Could you check a few things on this model? Use its own coordinates, in mm. A direction names the side the tool comes from. Coordinates: 2 decimals unless noted, no trailing zeros. Order: outer loops, then holes, each group sorted by start corner. A loop starts at its lowest first (then second) coordinate and runs counter-clockwise, first axis right, second up. Notation, with made-up numbers: M -8,-13.5 L -2,-13.5 A16 ccw -2,6.5 Z; hole C -15.75,32 d5. An arc over 180 degrees is marked long. Put each result on its own line as item: value. Start each with the question number.
```python
from build123d import *

# Parameters (mm, degrees)
F1_DEPTH      = 2.5
F2_R          = 1
F4_W          = 33
F4_H          = 5.5
F5_DEPTH      = 2
F5_DEPTH_BACK = 1


with BuildPart() as f1:
    # F0 (on Top) → F1 (new body)
    with BuildSketch(Plane.XY):
        Polygon((-23.6938069443, 68.3301911354), (-23.6938069443, -57.6698088646), (-10.9438069443, -57.6698088646), (-10.9438069443, -51.6698088646), (-7.9438069443, -51.6698088646), (-7.9438069443, -57.6698088646), (4.8061930557, -57.6698088646), (4.8061930557, 68.3301911354), align=None)
    extrude(amount=F1_DEPTH)

    # F2
    f2_edges = [f1.edges().sort_by_distance(p)[0] for p in [
        (-10.943807, -51.669809, 1.25),
        (-7.943807, -51.669809, 1.25),
    ]]
    fillet(f2_edges, radius=F2_R)

    # F4 (on face) → F5 (join, two sides)
    with BuildSketch(Plane(origin=(0, 67.8111465652, -5.9327065851), x_dir=(1, 0, 0), z_dir=(0, -0.9961946981, 0.0871557427))) as f5_sk:
        with Locations((-9.4438069443, 8.7053685605)):
            Rectangle(F4_W, F4_H)
    extrude(amount=-F5_DEPTH)
    extrude(f5_sk.sketch, amount=F5_DEPTH_BACK)


solid = f1.part
```
Item 1: If we section it at C-C on z = 4.15: Write out the boundary of the cut face in (x, y), then the cut area to 3 significant figures.
Item 2: I need wall thicknesses on probe 1 along Z at (x, y) = (-11, 40); probe 2 along X at (y, z) = (1.5, 1.4); probe 3 along Y at (x, z) = (-16, 3.4). Which ranges of each line are inside material? Lowest first, please.
Item 3: If we mould it in two halves opening along X, with no side actions, what happens to faces 4 (the flat face through (7.056, 69, 3)), 5 (the flat face through (-10, 6, 2.5)), 6 (the flat face through (-7.944, -55, 1))? For each: released by +X, released by -X, zero draft, split by the parting line, or undercut.
Item 4: For faces 1 (the flat face through (-10, 6, 0)), 2 (the flat face through (-23.694, 6, 1)), 3 (the flat face through (-10.944, -55, 1)), which set-ups out of +Z, -Z, +X, -X, +Y, -Y let a thin tool reach every point of the face, with its end or its side?
Item 5: If we section it at A-A on x = 3.5: Write out the boundary of the cut face in (y, z).
Item 6: For pin 1 Ø12 at (x, y) = (-12, -33) entering from +Z; pin 2 Ø2 at (y, z) = (-56.5, 1) entering from +X; pin 3 Ø0.8 at (y, z) = (-14.5, 2) entering from -X, each with a flat end and sliding along its axis, tell me the tip position at first contact or that it passes through.
Item 7: If we section it at B-B on y = 50: Write out the boundary of the cut face in (x, z), then the cut area to 4 significant figures.
Geometry check:
1. outline: M -25.94,67.69 L 7.06,67.69 L 7.06,70.7 L -25.94,70.7 Z
1. area: 99.4 mm²
2. probe 1: z = 0 to 2.5
2. probe 2: x = -23.69 to 4.81
2. probe 3: y = 67.62 to 70.64
3. face 4: released by +X
3. face 5: zero draft
3. face 6: undercut
4. face 1: -Z, +X, -X, -Y
4. face 2: +Z, -Z, -X, -Y
4. face 3: +Z, -Z, -Y
5. outline: M -57.67,0 L 68.33,0 L 70.32,-0.17 L 70.8,5.3 L 67.81,5.57 L 67.55,2.5 L -57.67,2.5 Z
6. pin 1: stops at z = 2.5
6. pin 2: stops at x = 4.81
6. pin 3: stops at x = -23.69
7. outline: M -23.69,0 L 4.81,0 L 4.81,2.5 L -23.69,2.5 Z
7. area: 71.25 mm²
